from build123d import *

# Parameters (mm, degrees)
SKETCH2_R           = 2
BOSS_EXTRUDE1_DEPTH = 20.32
SKETCH3_R           = 2
CUT_EXTRUDE1_DEPTH  = 6.35
SKETCH4_R           = 4.7625
BOSS_EXTRUDE2_DEPTH = 6.35
SKETCH5_R           = 2.8
CUT_EXTRUDE2_DEPTH  = 4.7
CHAMFER2_SIZE       = 2.54
CHAMFER2_SIZE2      = 0.447870531


with BuildPart() as part:
    # Sketch2 → Boss-Extrude1 (new body)
    with BuildSketch(Plane.XY):
        with BuildLine():
            ThreePointArc((0, 5.08), (-5.08, 0), (0, -5.08))
            Line((0, -5.08), (8.89, -5.08))
            Line((8.89, -5.08), (8.89, 5.08))
            Line((8.89, 5.08), (0, 5.08))
        make_face()
        Circle(SKETCH2_R, mode=Mode.SUBTRACT)
    extrude(amount=BOSS_EXTRUDE1_DEPTH)

    # Sketch3 → Cut-Extrude1 (cut, symmetric)
    with BuildSketch(Plane.XY.offset(10.16)):
        with BuildLine():
            ThreePointArc((0, 5.08), (-5.08, 0), (0, -5.08))
            ThreePointArc((0, -5.08), (2.090104165, -4.630104165), (3.81, -3.360104165))
            Line((3.81, -3.360104165), (3.81, 3.360104165))
            ThreePointArc((3.81, 3.360104165), (2.090104165, 4.630104165), (0, 5.08))
        make_face()
        Circle(SKETCH3_R, mode=Mode.SUBTRACT)
        with BuildLine():
            Line((3.81, 5.08), (0, 5.08))
            ThreePointArc((0, 5.08), (2.090104165, 4.630104165), (3.81, 3.360104165))
            Line((3.81, 3.360104165), (3.81, 5.08))
        make_face()
        with BuildLine():
            Line((0, -5.08), (3.81, -5.08))
            Line((3.81, -5.08), (3.81, -3.360104165))
            ThreePointArc((3.81, -3.360104165), (2.090104165, -4.630104165), (0, -5.08))
        make_face()
    extrude(amount=CUT_EXTRUDE1_DEPTH, both=True, mode=Mode.SUBTRACT)

    # Sketch4 → Boss-Extrude2 (add)
    with BuildSketch(Plane(origin=(8.89, 0, 0), x_dir=(0, 0, -1), z_dir=(1, 0, 0))):
        with Locations((-10.16, 0)):
            Circle(SKETCH4_R)
    extrude(amount=BOSS_EXTRUDE2_DEPTH)

    # Sketch5 → Cut-Extrude2 (cut)
    with BuildSketch(Plane(origin=(15.24, 0, 0), x_dir=(0, 0, -1), z_dir=(1, 0, 0))):
        with Locations((-10.16, 0)):
            Circle(SKETCH5_R)
    extrude(amount=-CUT_EXTRUDE2_DEPTH, mode=Mode.SUBTRACT)

    # Chamfer2
    chamfer2_edges = [part.edges().sort_by_distance(p)[0] for p in [
        (3.81, 5.08, 10.16),
        (3.81, -5.08, 10.16),
    ]]
    chamfer2_side = [part.faces().sort_by_distance(p)[0] for p in [
        (3.81, 0, 10.16),
    ]]
    chamfer(chamfer2_edges, length=CHAMFER2_SIZE, length2=CHAMFER2_SIZE2, reference=chamfer2_side[0])


solid = part.part
The listing builds one solid part. Answer for the finished solid, in the listing's coordinates (mm). A direction names the side the tool comes from. Give positions to 0.01 mm unless a question says otherwise; leave off trailing zeros. Write each loop counter-clockwise with the first axis right and the second up, starting at its lowest first coordinate (ties: lowest second). Pieces come first, ordered by that corner, then holes.
Item 1: Find the intervals of material crossed by line 1 along Z through (x, y) = (-3.75, -0.25); line 2 along Y through (x, z) = (14.15, 10.16); line 3 along Y through (x, z) = (10.75, 10.75), in increasing order.
Item 2: Flat-ended cylindrical pins translate along their axes: P1, Ø4, axis at y = 1, z = 9, coming from the -X side; P2, Ø1.7, axis at y = 1, z = 10.5, coming from the +X side; P3, Ø6, axis at y = 4, z = 3, coming from the -X side. Find the tip coordinate at first contact, or state that the pin passes through.
Item 3: Section D-D, the plane z = 10.16 is taken. Write down the section's boundary in (x, y), plus the area to 3 significant figures.
Item 4: Section C-C, the plane z = 2.25 is taken. Write down the section's boundary in (x, y).
Item 5: Determine the mould class of faces 1 (the flat face through (4.037, -3.828, 10.071)), 2 (the cylindrical face through (0, -2, 2)), 3 (the flat face through (3, 0, 0)) for opening direction Y: released by +Y, released by -Y, zero draft, split by the parting line, or undercut.
Item 6: Section B-B, the plane y = 0 is taken. Write down the section's boundary in (x, z), plus the area to 3 significant figures.
Item 7: Section A-A, the plane x = 2.75 is taken. Write down the section's boundary in (y, z).
Item 8: Which of the six approach directions +Z, -Z, +X, -X, +Y, -Y give full straight-line access (tool end or side, diameter ignored) to faces 4 (the flat face through (4.037, 3.828, 10.249)), 5 (the flat face through (8.89, -2.3, 5.5)), 6 (the flat face through (3.81, 0, 10))?
Completed:
1. line 1: z = 0 to 3.81, 16.51 to 20.32
1. line 2: y = -4.76 to -2.8, 2.8 to 4.76
1. line 3: y = -4.73 to -2.74, 2.74 to 4.73
2. P1: stops at x = 3.81
2. P2: stops at x = 10.54
2. P3: stops at x = -4.98
3. outline: (3.81, -2.54) - (4.26, -5.08) - (8.89, -5.08) - (8.89, -4.76) - (15.24, -4.76) - (15.24, -2.8) - (10.54, -2.8) - (10.54, 2.8) - (15.24, 2.8) - (15.24, 4.76) - (8.89, 4.76) - (8.89, 5.08) - (4.26, 5.08) - (3.81, 2.54) - close
3. area: 84.6 mm2
4. outline: (0, -5.08) - (8.89, -5.08) - (8.89, 5.08) - (0, 5.08) arc R5.08 ccw to start; hole circle Ø4 at (0, 0)
5. face 1: released by -Y
5. face 2: undercut
5. face 3: zero draft
6. outline: (-5.08, 0) - (-2, 0) - (-2, 3.81) - (-5.08, 3.81) - close; (-5.08, 16.51) - (-2, 16.51) - (-2, 20.32) - (-5.08, 20.32) - close; (2, 0) - (8.89, 0) - (8.89, 5.4) - (15.24, 5.4) - (15.24, 7.36) - (10.54, 7.36) - (10.54, 12.96) - (15.24, 12.96) - (15.24, 14.92) - (8.89, 14.92) - (8.89, 20.32) - (2, 20.32) - (2, 16.51) - (3.81, 16.51) - (3.81, 3.81) - (2, 3.81) - close
6. area: 175 mm2
7. outline: (-5.08, 0) - (5.08, 0) - (5.08, 3.81) - (-5.08, 3.81) - close; (-5.08, 16.51) - (5.08, 16.51) - (5.08, 20.32) - (-5.08, 20.32) - close
8. face 4: -X, +Y
8. face 5: +X
8. face 6: -X, +Y, -Y
